The listing builds one solid part. Answer for the finished solid, in the listing's coordinates (mm). A direction names the side the tool comes from. Give positions to 0.01 mm unless a question says otherwise; leave off trailing zeros. Loops run counter-clockwise (first coordinate to the right, second up) from the corner with the lowest first, then second, coordinate; pieces in that order, holes last. Notation, with made-up numbers: (8, 69.5) - (40, 69.5) arc R13 cw to (40, 85.5) - close; hole circle Ø11 at (62, 83.25). An arc over 180 degrees is marked (long way). One line per item, written item: value. Start each with the question number.
from build123d import *

# Parameters (mm, degrees)
EXTRUDE_1_DEPTH     = 2
SKETCH_2_W          = 42
SKETCH_2_H          = 2
EXTRUDE_2_DEPTH     = 25.3
SKETCH_3_W          = 8.5
SKETCH_3_H          = 2
EXTRUDE_3_DEPTH     = 25
FILLET_3_R          = 3
FILLET_4_R          = 3
FILLET_5_R          = 3
FILLET_6_R          = 3
FILLET_7_R          = 3
FILLET_8_R          = 3
FILLET_9_R          = 3
FILLET_10_R         = 3
FILLET_11_R         = 3
FILLET_12_R         = 3
SKETCH_5_R          = 1.5
SKETCH_5_R_2        = 4
SKETCH_5_R_3        = 1.9
CUT_EXTRUDE_5_DEPTH = 2
SKETCH_9_R          = 1.9
CUT_EXTRUDE_6_DEPTH = 2
SKETCH_10_R         = 1.5
CUT_EXTRUDE_7_DEPTH = 2
FILLET_13_R         = 3
FILLET_14_R         = 3
FILLET_15_R         = 3


with BuildPart() as part:
    # 草图1 → 凸台-拉伸1 (new body)
    with BuildSketch(Plane.XY):
        Polygon((0, 0), (42, 0), (42, -8.1), (50, -8.1), (50, -32.1), (41.5, -32.1), (41.5, -27.4), (39.4, -27.4), (39.4, -37.9), (2.6, -37.9), (2.6, -27.4), (0.5, -27.4), (0.5, -32.1), (-8, -32.1), (-8, -8.1), (0, -8.1), align=None)
    extrude(amount=EXTRUDE_1_DEPTH)

    # 草图2 → 凸台-拉伸2 (add)
    with BuildSketch(Plane(origin=(0, 0, 0), x_dir=(-1, 0, 0), z_dir=(0, 0, -1))):
        with Locations((-21, -1)):
            Rectangle(SKETCH_2_W, SKETCH_2_H)
    extrude(amount=EXTRUDE_2_DEPTH)

    # 草图3 → 凸台-拉伸3 (add)
    with BuildSketch(Plane(origin=(0, 0, 0), x_dir=(-1, 0, 0), z_dir=(0, 0, -1))):
        with Locations((-45.75, -31.1)):
            Rectangle(SKETCH_3_W, SKETCH_3_H)
        with Locations((3.75, -31.1)):
            Rectangle(SKETCH_3_W, SKETCH_3_H)
    extrude(amount=EXTRUDE_3_DEPTH)

    # 圆角3
    fillet_3_edges = [part.edges().sort_by_distance(p)[0] for p in [
        (42, -1, -25.3),
    ]]
    fillet(fillet_3_edges, radius=FILLET_3_R)

    # 圆角4
    fillet_4_edges = [part.edges().sort_by_distance(p)[0] for p in [
        (41.5, -31.1, -25),
    ]]
    fillet(fillet_4_edges, radius=FILLET_4_R)

    # 圆角5
    fillet_5_edges = [part.edges().sort_by_distance(p)[0] for p in [
        (0, -1, -25.3),
    ]]
    fillet(fillet_5_edges, radius=FILLET_5_R)

    # 圆角6
    fillet_6_edges = [part.edges().sort_by_distance(p)[0] for p in [
        (50, -31.1, -25),
    ]]
    fillet(fillet_6_edges, radius=FILLET_6_R)

    # 圆角7
    fillet_7_edges = [part.edges().sort_by_distance(p)[0] for p in [
        (-8, -31.1, -25),
    ]]
    fillet(fillet_7_edges, radius=FILLET_7_R)

    # 圆角8
    fillet_8_edges = [part.edges().sort_by_distance(p)[0] for p in [
        (0.5, -31.1, -25),
    ]]
    fillet(fillet_8_edges, radius=FILLET_8_R)

    # 圆角9
    fillet_9_edges = [part.edges().sort_by_distance(p)[0] for p in [
        (39.4, -37.9, 1),
    ]]
    fillet(fillet_9_edges, radius=FILLET_9_R)

    # 圆角10
    fillet_10_edges = [part.edges().sort_by_distance(p)[0] for p in [
        (2.6, -37.9, 1),
    ]]
    fillet(fillet_10_edges, radius=FILLET_10_R)

    # 圆角11
    fillet_11_edges = [part.edges().sort_by_distance(p)[0] for p in [
        (50, -8.1, 1),
    ]]
    fillet(fillet_11_edges, radius=FILLET_11_R)

    # 圆角12
    fillet_12_edges = [part.edges().sort_by_distance(p)[0] for p in [
        (-8, -8.1, 1),
    ]]
    fillet(fillet_12_edges, radius=FILLET_12_R)

    # 草图5 → 切除-拉伸5 (cut)
    with BuildSketch(Plane(origin=(0, 0, 0), x_dir=(-1, 0, 0), z_dir=(0, 0, -1))):
        with Locations((-32.8, -32.4)):
            Circle(SKETCH_5_R)
        with Locations((-32.8, -25.4)):
            Circle(SKETCH_5_R_2)
        with Locations((-25.8, -25.4)):
            Circle(SKETCH_5_R)
        with Locations((-32.8, -18.4)):
            Circle(SKETCH_5_R)
        with Locations((-39.8, -25.4)):
            Circle(SKETCH_5_R)
        with Locations((-21, -14.9)):
            Circle(SKETCH_5_R_2)
        with Locations((-14, -14.9)):
            Circle(SKETCH_5_R)
        with Locations((-21, -7.9)):
            Circle(SKETCH_5_R)
        with Locations((-21, -21.9)):
            Circle(SKETCH_5_R)
        with Locations((-44.86, -25)):
            Circle(SKETCH_5_R_3)
        with Locations((-44.86, -14.8)):
            Circle(SKETCH_5_R_3)
        with Locations((-28, -14.9)):
            Circle(SKETCH_5_R)
        with Locations((-9.2, -32.4)):
            Circle(SKETCH_5_R)
        with Locations((-9.2, -18.4)):
            Circle(SKETCH_5_R)
        with Locations((-16.2, -25.4)):
            Circle(SKETCH_5_R)
        with Locations((-9.2, -25.4)):
            Circle(SKETCH_5_R_2)
        with Locations((2.86, -25)):
            Circle(SKETCH_5_R_3)
        with Locations((2.86, -14.8)):
            Circle(SKETCH_5_R_3)
    extrude(amount=-CUT_EXTRUDE_5_DEPTH, mode=Mode.SUBTRACT)

    # 草图9 → 切除-拉伸6 (cut)
    with BuildSketch(Plane(origin=(0, -30.1, 0), x_dir=(1, 0, 0), z_dir=(0, 1, 0))):
        with Locations((44.85, 18.34)):
            Circle(SKETCH_9_R)
        with Locations((44.85, 8.54)):
            Circle(SKETCH_9_R)
        with Locations((-3.15, 8.54)):
            Circle(SKETCH_9_R)
        with Locations((-3.15, 18.34)):
            Circle(SKETCH_9_R)
    extrude(amount=-CUT_EXTRUDE_6_DEPTH, mode=Mode.SUBTRACT)

    # 草图10 → 切除-拉伸7 (cut)
    with BuildSketch(Plane.XZ.offset(2)):
        with Locations((10.6, -20.5)):
            Circle(SKETCH_10_R)
        with Locations((10.6, -13.5)):
            Circle(SKETCH_10_R)
        with Locations((10.6, -6.5)):
            Circle(SKETCH_10_R)
        with Locations((17.6, -13.5)):
            Circle(SKETCH_10_R)
        with Locations((3.6, -13.5)):
            Circle(SKETCH_10_R)
        with Locations((31.4, -20.5)):
            Circle(SKETCH_10_R)
        with Locations((24.4, -13.5)):
            Circle(SKETCH_10_R)
        with Locations((31.4, -13.5)):
            Circle(SKETCH_10_R)
        with Locations((38.4, -13.5)):
            Circle(SKETCH_10_R)
        with Locations((31.4, -6.5)):
            Circle(SKETCH_10_R)
    extrude(amount=-CUT_EXTRUDE_7_DEPTH, mode=Mode.SUBTRACT)

    # 圆角13
    fillet_13_edges = [part.edges().sort_by_distance(p)[0] for p in [
        (21, 0, 2),
    ]]
    fillet(fillet_13_edges, radius=FILLET_13_R)

    # 圆角14
    fillet_14_edges = [part.edges().sort_by_distance(p)[0] for p in [
        (45.75, -32.1, 2),
    ]]
    fillet(fillet_14_edges, radius=FILLET_14_R)

    # 圆角15
    fillet_15_edges = [part.edges().sort_by_distance(p)[0] for p in [
        (-3.75, -32.1, 2),
    ]]
    fillet(fillet_15_edges, radius=FILLET_15_R)


solid = part.part
1. A cutting plane is placed at C-C (x = 40.5). Determine the outline of the cut face in (y, z), plus the area to 3 significant figures.
2. A cutting plane is placed at D-D (x = -3.15). Determine the outline of the cut face in (y, z), plus the area to 3 significant figures.
3. A cutting plane is placed at B-B (y = -33). Determine the outline of the cut face in (x, z).
4. A cutting plane is placed at A-A (z = -2.5). Determine the outline of the cut face in (x, y).
5. Determine the mould class of faces 1 (the flat face through (21, -37.9, 1)), 2 (the cylindrical face through (-7.1, -8.96, 1.01)), 3 (the cylindrical face through (7.814, -32.975, 0.986)), 4 (the cylindrical face through (29.11, -13.89, 0.99)) for opening direction Y: released by +Y, released by -Y, zero draft, split by the parting line, or undercut.
6. Find the intervals of material crossed by L1, parallel to X at y = -30.55, z = -8.54; L2, parallel to Y at x = -3.5, z = -4.5; L3, parallel to Z at x = 24.5, y = -34, in increasing order. Write a range as [from, to].
7. Flat-ended cylindrical pins translate along their axes: pin 1 (7 mm diameter, centred on x = -4, z = -17, fed in from -Y); pin 2 (4.5 mm diameter, centred on x = 44.86, y = -14.8, fed in from -Z); pin 3 (3 mm diameter, centred on x = 33, z = -4, fed in from -Y); pin 4 (5 mm diameter, centred on x = 21, y = -14.9, fed in from +Z). Find the tip coordinate at first contact, or state that the pin passes through.
8. For faces 5 (the flat face through (2.6, -31, 1)), 6 (the cylindrical face through (25.995, -23.913, 0.986)), 7 (the cylindrical face through (42.36, -31.09, -24.1)), determine the directions among +Z, -Z, +X, -X, +Y, -Y from which every point of the face is accessible in a straight line to the end or side of a thin tool.
Results below:
1. outline: (-27.4, 0) - (-26.73, 0) - (-26.73, 2) - (-27.4, 2) - close; (-24.07, 0) - (-2, 0) - (-2, -24.9) - (0, -24.9) - (0, -1) arc R3 ccw to (-3, 2) - (-24.07, 2) - close
1. area: 97.4 mm^2
2. outline: (-32.1, -25) - (-30.1, -25) - (-30.1, -20.24) - (-32.1, -20.24) - close; (-32.1, -16.44) - (-30.1, -16.44) - (-30.1, -10.44) - (-32.1, -10.44) - close; (-32.1, -6.64) - (-30.1, -6.64) - (-30.1, 0) - (-26.88, 0) - (-26.88, 2) - (-29.1, 2) arc R3 ccw to (-32.1, -1) - close; (-23.12, 0) - (-16.68, 0) - (-16.68, 2) - (-23.12, 2) - close; (-12.92, 0) - (-8.1, 0) - (-8.1, 2) - (-12.92, 2) - close
2. area: 65.8 mm^2
3. outline: (2.6, 0) - (7.83, 0) - (7.83, 2) - (2.6, 2) - close; (10.57, 0) - (31.43, 0) - (31.43, 2) - (10.57, 2) - close; (34.17, 0) - (39.4, 0) - (39.4, 2) - (34.17, 2) - close
4. outline: (-8, -32.1) - (0.5, -32.1) - (0.5, -30.1) - (-8, -30.1) - close; (0, -2) - (42, -2) - (42, 0) - (0, 0) - close; (41.5, -32.1) - (50, -32.1) - (50, -30.1) - (41.5, -30.1) - close
5. face 1: released by -Y
5. face 2: released by +Y
5. face 3: undercut
5. face 4: undercut
6. L1: x = [-8, -5.05], [-1.25, 0.5], [41.5, 42.95], [46.75, 50]
6. L2: y = [-32.1, -30.1]
6. L3: z = [0, 2]
7. pin 1: stops at y = -32.1
7. pin 2: stops at z = 0
7. pin 3: stops at y = -2
7. pin 4: passes through
8. face 5: +Z, -Z, -Y
8. face 6: +Z, -Z
8. face 7: -Z, -Y
